from build123d import *

# Parameters (mm, degrees)
CHAMFER_1_SIZE = 0.2


with BuildPart() as part:
    # Sketch 2 → Revolve 539 (revolve)
    with BuildSketch(Plane.XY, mode=Mode.PRIVATE) as revolve_539_sk:
        with BuildLine():
            Line((0, 0), (7.6, 0))
            Line((7.6, 0), (7.6, 1))
            Line((7.6, 1), (1.7, 1))
            ThreePointArc((1.7, 1), (1.629289322, 1.029289322), (1.6, 1.1))
            Line((1.6, 1.1), (1.6, 2))
            Line((1.6, 2), (1.1, 2))
            ThreePointArc((1.1, 2), (0.293143234, 1.141271221), (0, 0))
        make_face()
    revolve(revolve_539_sk.sketch.rotate(Axis((-1.331757704, 0, 0), (1, 0, 0)), 90), axis=Axis((-1.331757704, 0, 0), (1, 0, 0)))

    # Sketch 5 → Loft 1 section 0
    with BuildSketch(Plane(origin=(0, 0, 0), x_dir=(0, 0, -1), z_dir=(1, 0, 0)), mode=Mode.PRIVATE) as loft_1_s0:
        with BuildLine():
            Line((0.25, 0.95), (-0.25, 0.95))
            Line((-0.25, 0.95), (-0.25, -0.95))
            Line((-0.25, -0.95), (0.25, -0.95))
            Line((0.25, -0.95), (0.25, 0.95))
        make_face()
    loft_1 = loft([Vertex(1.2, 0, 0), loft_1_s0.sketch], mode=Mode.SUBTRACT)

    # Mirror 1: Loft 1 across plane
    add(loft_1.mirror(Plane(origin=(0, 0, 0), x_dir=(0, 0.7071067811865462, 0.7071067811865488), z_dir=(0, -0.7071067811865488, 0.7071067811865462))), mode=Mode.SUBTRACT)

    # Chamfer 1
    chamfer_1_edges = [part.edges().sort_by_distance(p)[0] for p in [
        (7.6, 0, -1),
    ]]
    chamfer(chamfer_1_edges, length=CHAMFER_1_SIZE)


solid = part.part
Read the model definition and answer for the solid it produces. Units are mm, in the model's axes. A direction names the side the tool comes from. Round coordinates to 2 decimals unless told otherwise and drop trailing zeros. Write each loop counter-clockwise with the first axis right and the second up, starting at its lowest first coordinate (ties: lowest second). Pieces come first, ordered by that corner, then holes. Notation, with made-up numbers: (13, 63.25) - (58, 63.25) arc R21 ccw to (58, 84.25) - close; hole circle Ø9 at (28, -6). An arc over 180 degrees is marked (long way). One line per question, with ' | ' between items. Start each with the question number.
1. This flat-tipped pin is pushed along its axis until it touches: pin 1 (1 mm diameter, centred on x = 3, z = 0.5, fed in from -Y). Where does it stop, or does it pass through?
2. Section A-A (x = 7) is taken. Determine the outline of the cut face in (y, z), and give its area (3 significant figures).
3. Find the intervals of material crossed by probe 1 along Z at (x, y) = (6.5, -0.05); probe 2 along Y at (x, z) = (5.5, 0.2); probe 3 along X at (y, z) = (1.2, 1.35), in increasing order. Write a range as [from, to].
4. For faces 1 (the face through (1.6, 1, -1)), 2 (the face through (0.474, -0.315, 0.151)), 3 (the face through (1.346, 1.952, -0.434)), determine the directions among +Z, -Z, +X, -X, +Y, -Y from which every point of the face is accessible in a straight line to the end or side of a thin tool.
5. Section C-C (z = 1.4) is taken. Determine the outline of the cut face in (x, y), and give its area (3 significant figures).
6. For a pull along Y with two mould halves and no side action, classify faces 4 (the face through (7.6, 0, 0)), 5 (the face through (0.474, 0.151, 0.326)), 6 (the face through (5, 1, 0)) as +Y half, -Y half, draft (parallel to the pull), parting line (faces both ways), or undercut.
7. Section B-B (y = -1.3) is taken. Determine the outline of the cut face in (x, z).
Filled in:
1) pin 1: y = -1
2) outline: circle Ø2 at (0, 0) | area: 3.14 mm²
3) probe 1: [-1, 1] | probe 2: [-0.98, 0.98] | probe 3: [0.84, 1.6]
4) face 1: +X | face 2: -X | face 3: +X, -X
5) outline: (1.1, -1.43) - (1.6, -1.43) - (1.6, 1.43) - (1.1, 1.43) arc R1.91 ccw to start | area: 2.70 mm²
6) face 4: draft | face 5: undercut | face 6: parting line
7) outline: (1.1, -1.52) - (1.6, -1.52) - (1.6, 1.52) - (1.1, 1.52) arc R1.98 ccw to start
